Autodesk Inventor part; units mm, degrees
ref_plane "YZ Plane" through (0, 0, 0) normal (1, 0, 0) x (0, 1, 0)
ref_plane "XZ Plane" through (0, 0, 0) normal (0, 1, 0) x (-1, 0, 0)
ref_plane "XY Plane" through (0, 0, 0) normal (0, 0, 1) x (1, 0, 0)
sketch "Эскиз1" plane through (0, 0, 0) normal (0, 0, 1) x (1, 0, 0)
  arc A0 (-15, 0) -> (0, -15) centre (0, 0) ccw
  line L0 (-15, 0) -> (0, 0)
  line L1 (0, 0) -> (0, -15)
  dimension "d0" = 30
extrude "Выдавливание1" add sketch "Эскиз1" along normal blind 97
fillet "Сопряжение1" radius 15 1 edges at (-10.6066, -10.6066, 0)
sketch "Эскиз2" plane through (0, 0, 97) normal (0, 0, 1) x (1, 0, 0)
  circle A0 centre (-5, -5) radius 1.55
  line L0 (0, 0) -> (-15, 0)
  line L1 (0, -15) -> (0, 0)
  dimension "d4" = 3.1
  dimension "d5" = 5
  dimension "d6" = 5
extrude "Выдавливание2" cut sketch "Эскиз2" against normal blind 7
properties part number "уголок насу"
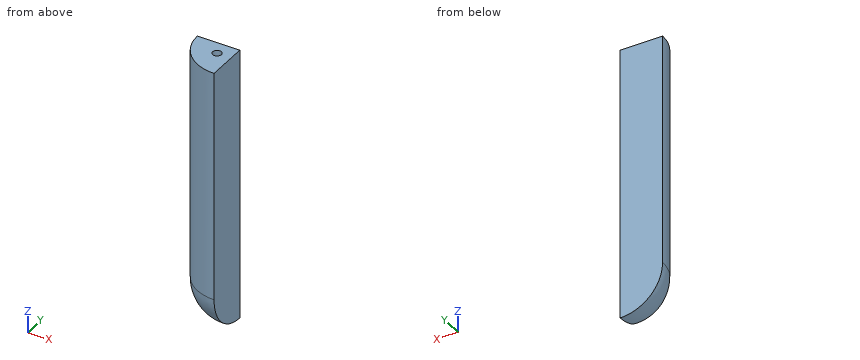
Part model, mm, in its own coordinate system. Coordinates: 2 decimals unless noted, no trailing zeros. Order: outer loops, then holes, each group sorted by start corner. A loop starts at its lowest first (then second) coordinate and runs counter-clockwise, first axis right, second up.
(1) Pin check, flat tips, straight feed: pin 1 Ø1 at (x, y) = (-1.5, -13) entering from -Z; pin 2 Ø5 at (y, z) = (-11.5, 43) entering from +X; pin 3 Ø3 at (x, y) = (-5, -5) entering from -Z; pin 4 Ø1.5 at (x, y) = (-11, -9.5) entering from -Z. Stop position of each tip, or through.
Check sheet entries:
pin 1: stops at z = 6.84
pin 2: stops at x = 0
pin 3: stops at z = 1.07
pin 4: stops at z = 9.08
(2) Probe L1, parallel to Y at x = -0.75, z = 35.5; L2, parallel to Y at x = -5, z = 95.25; L3, parallel to X at y = -13.5, z = 25.5. List the from-to ranges inside material, lowest first.
Check sheet entries:
L1: y = -14.98 to 0
L2: y = -14.14 to -6.55, -3.45 to 0
L3: x = -6.54 to 0
(3) Slice it at A-A, the plane z = 62. Write the cut outline in (x, y), and give its area (3 significant figures).
Check sheet entries:
outline: (-15, 0) arc R15 ccw to (0, -15) - (0, 0) - close
area: 177 mm2
